Can you work these out from the model? Positions are in its coordinate system, mm. Face numbers are marked on the shaded views. A direction names the side the tool comes from. Give positions to 0.01 mm unless a question says otherwise; leave off trailing zeros. Order: outer loops, then holes, each group sorted by start corner. A loop starts at its lowest first (then second) coordinate and runs counter-clockwise, first axis right, second up. Notation, with made-up numbers: M 34.25,73.25 L 56.25,73.25 A25 ccw 56.25,107.25 Z; hole C 24,5 d9. An arc over 180 degrees is marked long. Use a Markdown table: item, result. Add a question column.
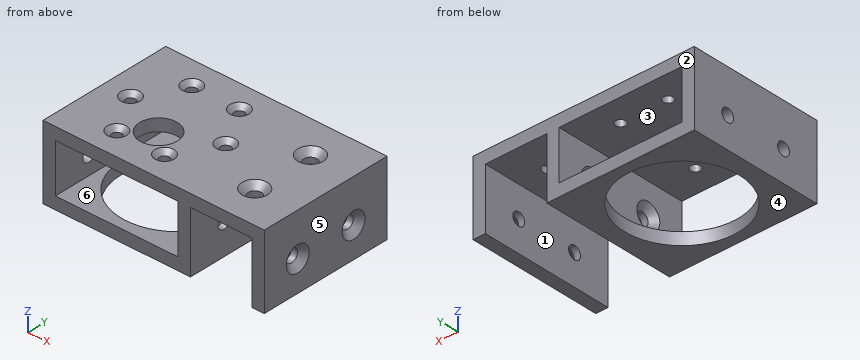
from build123d import *

# Parameters (mm, degrees)
SKETCH1_W           = 40
SKETCH1_H           = 16
BOSS_EXTRUDE1_DEPTH = 44
CUT_EXTRUDE1_REACH  = 86.475
SKETCH2_R           = 18.625
CUT_EXTRUDE2_REACH  = 86.475
SKETCH3_R           = 6.125
SKETCH3_R_2         = 1.625
SKETCH4_R           = 2.125
CUT_EXTRUDE3_DEPTH  = 87.717933555
SKETCH5_R           = 2.125
CUT_EXTRUDE4_DEPTH  = 85.474848328
CHAMFER1_SIZE       = 2
CHAMFER2_SIZE       = 1.5


with BuildPart() as part:
    # Sketch1 → Boss-Extrude1 (new body)
    with BuildSketch(Plane(origin=(0, 0, 0), x_dir=(1, 0, 0), z_dir=(0, 1, 0))):
        Polygon((4, 20), (0, 20), (0, 0), (-20, 0), (-20, 20), (-24, 20), (-68, 20), (-68, 16), (-68, 0), (-68, -4), (-24, -4), (4, -4), align=None)
        with Locations((-44, 8)):
            Rectangle(SKETCH1_W, SKETCH1_H, mode=Mode.SUBTRACT)
    extrude(amount=BOSS_EXTRUDE1_DEPTH)

    # Sketch2 → Cut-Extrude1 (cut, up to next)
    with BuildSketch(Plane(origin=(0, 0, -20), x_dir=(-1, 0, 0), z_dir=(0, 0, -1)), mode=Mode.PRIVATE) as cut_extrude1_sk1:
        with Locations((44, 22)):
            Circle(SKETCH2_R)
    cut_extrude1_tool1 = extrude(cut_extrude1_sk1.sketch, amount=-CUT_EXTRUDE1_REACH, mode=Mode.PRIVATE) & part.part
    add(cut_extrude1_tool1.solids().sort_by_distance((-44, 22, -20))[0], mode=Mode.SUBTRACT)

    # Sketch3 → Cut-Extrude2 (cut, up to next)
    with BuildSketch(Plane.XY.offset(4), mode=Mode.PRIVATE) as cut_extrude2_sk1:
        with Locations((-44, 15)):
            Circle(SKETCH3_R)
    cut_extrude2_tool1 = extrude(cut_extrude2_sk1.sketch, amount=-CUT_EXTRUDE2_REACH, mode=Mode.PRIVATE) & part.part
    # Sketch3 → Cut-Extrude2 (cut, up to next)
    with BuildSketch(Plane.XY.offset(4), mode=Mode.PRIVATE) as cut_extrude2_sk2:
        with Locations((-51.75, 35.423393759)):
            Circle(SKETCH3_R_2)
    cut_extrude2_tool2 = extrude(cut_extrude2_sk2.sketch, amount=-CUT_EXTRUDE2_REACH, mode=Mode.PRIVATE) & part.part
    # Sketch3 → Cut-Extrude2 (cut, up to next)
    with BuildSketch(Plane.XY.offset(4), mode=Mode.PRIVATE) as cut_extrude2_sk3:
        with Locations((-36.25, 35.423393759)):
            Circle(SKETCH3_R_2)
    cut_extrude2_tool3 = extrude(cut_extrude2_sk3.sketch, amount=-CUT_EXTRUDE2_REACH, mode=Mode.PRIVATE) & part.part
    # Sketch3 → Cut-Extrude2 (cut, up to next)
    with BuildSketch(Plane.XY.offset(4), mode=Mode.PRIVATE) as cut_extrude2_sk4:
        with Locations((-28.5, 22)):
            Circle(SKETCH3_R_2)
    cut_extrude2_tool4 = extrude(cut_extrude2_sk4.sketch, amount=-CUT_EXTRUDE2_REACH, mode=Mode.PRIVATE) & part.part
    # Sketch3 → Cut-Extrude2 (cut, up to next)
    with BuildSketch(Plane.XY.offset(4), mode=Mode.PRIVATE) as cut_extrude2_sk5:
        with Locations((-36.25, 8.576606241)):
            Circle(SKETCH3_R_2)
    cut_extrude2_tool5 = extrude(cut_extrude2_sk5.sketch, amount=-CUT_EXTRUDE2_REACH, mode=Mode.PRIVATE) & part.part
    # Sketch3 → Cut-Extrude2 (cut, up to next)
    with BuildSketch(Plane.XY.offset(4), mode=Mode.PRIVATE) as cut_extrude2_sk6:
        with Locations((-51.75, 8.576606241)):
            Circle(SKETCH3_R_2)
    cut_extrude2_tool6 = extrude(cut_extrude2_sk6.sketch, amount=-CUT_EXTRUDE2_REACH, mode=Mode.PRIVATE) & part.part
    # Sketch3 → Cut-Extrude2 (cut, up to next)
    with BuildSketch(Plane.XY.offset(4), mode=Mode.PRIVATE) as cut_extrude2_sk7:
        with Locations((-59.5, 22)):
            Circle(SKETCH3_R_2)
    cut_extrude2_tool7 = extrude(cut_extrude2_sk7.sketch, amount=-CUT_EXTRUDE2_REACH, mode=Mode.PRIVATE) & part.part
    add(cut_extrude2_tool1.solids().sort_by_distance((-44, 15, 4))[0], mode=Mode.SUBTRACT)
    add(cut_extrude2_tool2.solids().sort_by_distance((-51.75, 35.423394, 4))[0], mode=Mode.SUBTRACT)
    add(cut_extrude2_tool3.solids().sort_by_distance((-36.25, 35.423394, 4))[0], mode=Mode.SUBTRACT)
    add(cut_extrude2_tool4.solids().sort_by_distance((-28.5, 22, 4))[0], mode=Mode.SUBTRACT)
    add(cut_extrude2_tool5.solids().sort_by_distance((-36.25, 8.576606, 4))[0], mode=Mode.SUBTRACT)
    add(cut_extrude2_tool6.solids().sort_by_distance((-51.75, 8.576606, 4))[0], mode=Mode.SUBTRACT)
    add(cut_extrude2_tool7.solids().sort_by_distance((-59.5, 22, 4))[0], mode=Mode.SUBTRACT)

    # Sketch4 → Cut-Extrude3 (cut, through all)
    with BuildSketch(Plane(origin=(4, 0, 0), x_dir=(0, 0, -1), z_dir=(1, 0, 0))):
        with Locations((10, 32)):
            Circle(SKETCH4_R)
        with Locations((10, 12)):
            Circle(SKETCH4_R)
    extrude(amount=-CUT_EXTRUDE3_DEPTH, mode=Mode.SUBTRACT)

    # Sketch5 → Cut-Extrude4 (cut, through all)
    with BuildSketch(Plane.XY.offset(4)):
        with Locations((-10, 32)):
            Circle(SKETCH5_R)
        with Locations((-10, 12)):
            Circle(SKETCH5_R)
    extrude(amount=-CUT_EXTRUDE4_DEPTH, mode=Mode.SUBTRACT)

    # Chamfer1
    chamfer1_edges = [part.edges().sort_by_distance(p)[0] for p in [
        (-12.125, 32, 4),
        (-12.125, 12, 4),
        (-24, 32, -7.875),
        (4, 32, -7.875),
        (-24, 12, -7.875),
        (4, 12, -7.875),
    ]]
    chamfer(chamfer1_edges, length=CHAMFER1_SIZE)

    # Chamfer2
    chamfer2_edges = [part.edges().sort_by_distance(p)[0] for p in [
        (-53.375, 35.423393759, 4),
        (-37.875, 35.423393759, 4),
        (-30.125, 22, 4),
        (-37.875, 8.576606241, 4),
        (-53.375, 8.576606241, 4),
        (-61.125, 22, 4),
    ]]
    chamfer(chamfer2_edges, length=CHAMFER2_SIZE)


solid = part.part
1. On a 3-axis mill with a long thin cutter (end or side, diameter ignored), from which of +Z, -Z, +X, -X, +Y, -Y can I reach the whole of each face in a straight line? I mean the marked faces 1, 2 and 3. Say none if no direction works.
2. I need wall thicknesses on L1, parallel to Y at x = -36.25, z = 0.9; L2, parallel to X at y = 41, z = -9; L3, parallel to Y at x = 0.85, z = -10 (3 decimals). Which ranges of each line are inside material? Lowest first, please. Write a range as [from, to].
3. Will these pins go through, and if not, where does the flat tip stop? pin 1 (5 mm diameter, centred on y = 12, z = -10, fed in from +X) (3 decimals); pin 2 (20 mm diameter, centred on x = -43.5, y = 18, fed in from -Z); pin 3 (5 mm diameter, centred on x = -51.75, y = 8.58, fed in from +Z).
4. If we section it at D-D, the plane x = -51.75: List the corners of the cut face in (y, z) for me.
5. If we section it at A-A, the plane x = -44: List the corners of the cut face in (y, z) for me (3 decimals), then the cut area to 3 significant figures.
6. If we section it at B-B, the plane x = -21: List the corners of the cut face in (y, z) for me (3 decimals), then the cut area to 3 significant figures.
7. If we section it at C-C, the plane z = -13: State how many separate pieces and enclosed holes the cut face has, then the cut area to 3 significant figures.
8. We'd pull the mould along Z, two halves only. Please class the marked faces 4, 5 and 6: +Z half, -Z half, draft (parallel to the pull), parting line (faces both ways), or undercut.
Geometry results:
| question | item | result |
|---|---|---|
| 1 | face 1 | -Z, +Y, -Y |
| 1 | face 2 | +Z, -Z, +X, -X, +Y |
| 1 | face 3 | +Y, -Y |
| 2 | L1 | y = [0, 6.95], [10.2, 33.8], [37.05, 44] |
| 2 | L2 | x = [-68, -64], [-24, -20], [0, 4] |
| 2 | L3 | y = [0, 9.875], [14.125, 29.875], [34.125, 44] |
| 3 | pin 1 | stops at x = 2.375 |
| 3 | pin 2 | stops at z = 0 |
| 3 | pin 3 | stops at z = 3.38 |
| 4 | outline | M 0,-20 L 5.06,-20 L 5.06,-16 L 0,-16 Z; M 0,0 L 6.95,0 L 6.95,2.5 L 5.45,4 L 0,4 Z; M 10.2,0 L 33.8,0 L 33.8,2.5 L 32.3,4 L 11.7,4 L 10.2,2.5 Z; M 37.05,0 L 44,0 L 44,4 L 38.55,4 L 37.05,2.5 Z; M 38.94,-20 L 44,-20 L 44,-16 L 38.94,-16 Z |
| 5 | outline | M 0,-20 L 3.375,-20 L 3.375,-16 L 0,-16 Z; M 0,0 L 8.875,0 L 8.875,4 L 0,4 Z; M 21.125,0 L 44,0 L 44,4 L 21.125,4 Z; M 40.625,-20 L 44,-20 L 44,-16 L 40.625,-16 Z |
| 5 | area | 154 mm^2 |
| 6 | outline | M 0,-20 L 44,-20 L 44,4 L 0,4 Z; hole C 12,-10 d4.25; hole C 32,-10 d4.25 |
| 6 | area | 1,030 mm^2 |
| 7 | separate pieces | 3 |
| 7 | enclosed holes | 0 |
| 7 | area | 512 mm^2 |
| 8 | face 4 | -Z half |
| 8 | face 5 | draft |
| 8 | face 6 | undercut |
